Could you check a few things on this model? Use its own coordinates, in mm. Face numbers are marked on the shaded views. A direction names the side the tool comes from. Coordinates: 2 decimals unless noted, no trailing zeros. Loops run counter-clockwise (first coordinate to the right, second up) from the corner with the lowest first, then second, coordinate; pieces in that order, holes last. Notation, with made-up numbers: (-9, 73.25) - (47, 73.25) arc R12 cw to (47, 90.25) - close; hole circle Ø2 at (85, -36.5). An arc over 180 degrees is marked (long way). One line per item, written item: value. Start each with the question number.
(1) If we mould it in two halves opening along X, with no side actions, what happens to the marked faces 3, 4, 5 and 6? For each: pulls with the +X half, pulls with the -X half, needs draft (parallel to the pull), parting line crosses it, or undercut.
(2) On a 3-axis mill with a long thin cutter (end or side, diameter ignored), from which of +Z, -Z, +X, -X, +Y, -Y can I reach the whole of each face in a straight line? I mean the marked faces 1 and 2. Say none if no direction works.
(3) I'm going to push a flat-ended pin straight in: P1, Ø1, axis at x = 16, z = 2.5, coming from the -Y side. Where does the tip first touch, or does it pass through?
(4) If I drill on line 1 along X through (y, z) = (1.5, 9.25); line 2 along Y through (x, z) = (18.5, 3); line 3 along Z through (x, y) = (11, -2.5), over which ranges is the centre line in solid material (lowest first)? Write a range as from..to.
(5) If we section it at C-C on x = 17.75: Write out the boundary of the cut face in (y, z), then the cut area to 3 significant figures.
(6) If we section it at B-B on y = 0: Write out the boundary of the cut face in (x, z).
(7) If we section it at A-A on z = 3: Write out the boundary of the cut face in (x, y).
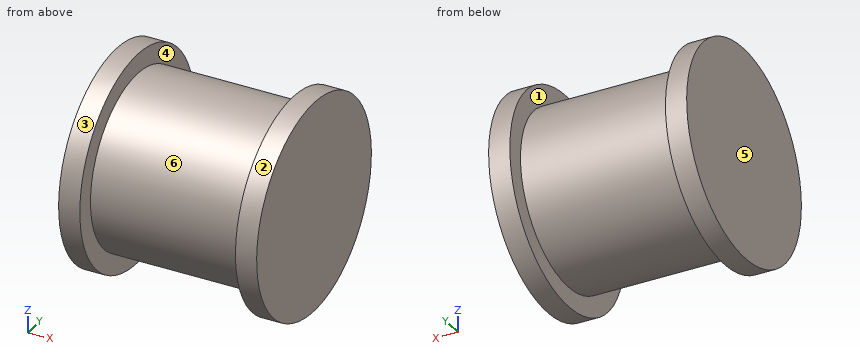
```python
from build123d import *

# Parameters (mm, degrees)
CYLINDER012_R     = 7.5
CYLINDER012_DEPTH = 1.5
CYLINDER011_R     = 6.11
CYLINDER011_DEPTH = 11
CYLINDER013_R     = 7.5
CYLINDER013_DEPTH = 1.5


with BuildPart() as cylinder012:
    # Cylinder012 → Cylinder012 (new body)
    with BuildSketch(Plane.ZY.offset(5.5)):
        Circle(CYLINDER012_R)
    extrude(amount=CYLINDER012_DEPTH)


with BuildPart() as cylinder011:
    # Cylinder011 → Cylinder011 (new body)
    with BuildSketch(Plane.ZY.offset(-5.5)):
        Circle(CYLINDER011_R)
    extrude(amount=CYLINDER011_DEPTH)


with BuildPart() as f_20t_9mm_pulley:
    # Cylinder013 → Cylinder013 (new body)
    with BuildSketch(Plane.ZY.offset(-7)):
        Circle(CYLINDER013_R)
    extrude(amount=CYLINDER013_DEPTH)

    # Fusion013005011003: union Cylinder012, Cylinder011
    add(cylinder012.part)
    add(cylinder011.part)


with BuildPart() as f_20t_9mm_pulley_1:
    # Fusion013005011003 placement: moved
    add(f_20t_9mm_pulley.part.moved(Location((15.5, 0, 3))))


solid = f_20t_9mm_pulley_1.part
```
Values:
1. face 3: needs draft
1. face 4: undercut
1. face 5: pulls with the -X half
1. face 6: undercut
2. face 1: none
2. face 2: +X, -X
3. P1: stops at y = -6.11
4. line 1: x = 8.5..10, 21..22.5
4. line 2: y = -6.11..6.11
4. line 3: z = -2.58..8.58
5. outline: circle Ø12.22 at (0, 3)
5. area: 117 mm2
6. outline: (8.5, -4.5) - (10, -4.5) - (10, -3.11) - (21, -3.11) - (21, -4.5) - (22.5, -4.5) - (22.5, 10.5) - (21, 10.5) - (21, 9.11) - (10, 9.11) - (10, 10.5) - (8.5, 10.5) - close
7. outline: (8.5, -7.5) - (10, -7.5) - (10, -6.11) - (21, -6.11) - (21, -7.5) - (22.5, -7.5) - (22.5, 7.5) - (21, 7.5) - (21, 6.11) - (10, 6.11) - (10, 7.5) - (8.5, 7.5) - close
